The listing builds one solid part. Answer for the finished solid, in the listing's coordinates (mm). Face numbers are marked on the shaded views. Round coordinates to 2 decimals unless told otherwise and drop trailing zeros. Write each loop counter-clockwise with the first axis right and the second up, starting at its lowest first coordinate (ties: lowest second). Pieces come first, ordered by that corner, then holes. Notation, with made-up numbers: (-12, 34.25) - (34, 34.25) arc R6 ccw to (34, 44.25) - close; hole circle Ø1 at (-9.75, -8). An arc over 180 degrees is marked (long way). Answer as CSV lines item,"result". Start each with the question number.
Item 1: A cutting plane is placed at B-B on y = 0. Determine the outline of the cut face in (x, z), and give its area (3 significant figures).
Item 2: Straight lines are drawn through the part: line 1 along X through (y, z) = (0, 13.25); line 2 along Y through (x, z) = (25.5, -5); line 3 along Y through (x, z) = (-10.5, 2). For each, find the intervals that lie inside material, in ascending order. Write a range as [from, to].
Item 3: Flat-ended cylindrical pins translate along their axes: pin 1 (1.4 mm diameter, centred on x = -12, z = 9, fed in from +Y); pin 2 (3 mm diameter, centred on x = 29.337, y = 0, fed in from -Z); pin 3 (1 mm diameter, centred on x = -6, y = 12.5, fed in from -Z). Find the tip coordinate at first contact, or state that the pin passes through.
Item 4: A cutting plane is placed at A-A on z = 0. Determine the outline of the cut face in (x, y), and give its area (3 significant figures).
Item 5: For a pull along Z with two mould halves and no side action, classify the marked faces 1, 2 and 3 as pulls with the +Z half, pulls with the -Z half, needs draft (parallel to the pull), parting line crosses it, or undercut.
```python
from build123d import *

# Parameters (mm, degrees)
F0_R     = 19.05
F1_DEPTH = 42.037
F4_D     = 3.7973
F4_DEPTH = 12
F4_START = 0.0948523
F4_TIP   = 1.1408240143
F5_SIZE  = 1.524


with BuildPart() as f1:
    # F0 (on Right) → F1 (new body, symmetric)
    with BuildSketch(Plane.YZ):
        Circle(F0_R)
        with BuildLine():
            ThreePointArc((2.38125, 7.5718924112), (0, -7.9375), (-2.38125, 7.5718924112))
            Line((-2.38125, 7.5718924112), (-2.38125, 10.31875))
            Line((-2.38125, 10.31875), (2.38125, 10.31875))
            Line((2.38125, 10.31875), (2.38125, 7.5718924112))
        make_face(mode=Mode.SUBTRACT)
    extrude(amount=F1_DEPTH, both=True)

    # F4
    # its depths count from where the whole tool has entered the part; down to there all is cleared
    with Locations(Plane.XY.offset(19.05).offset(-F4_START)):
        with Locations((29.337, 0), (-29.337, 0)):
            Hole(F4_D / 2, depth=F4_DEPTH)
            with Locations((0, 0, -(F4_DEPTH + F4_TIP / 2))):  # 118° drill point
                Cone(0, F4_D / 2, F4_TIP, mode=Mode.SUBTRACT)

    # F5
    f5_edges = [f1.edges().sort_by_distance(p)[0] for p in [
        (42.037, -19.05, 0),
        (-42.037, -19.05, 0),
    ]]
    chamfer(f5_edges, length=F5_SIZE)


solid = f1.part
```
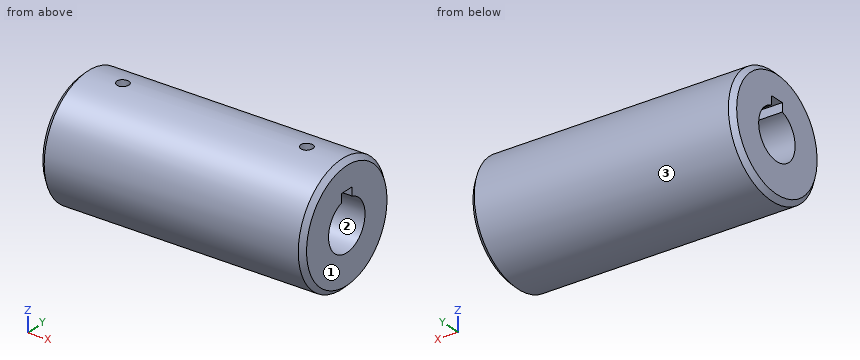
Geometry says:
1,outline,"(-42.04, -17.53) - (-40.51, -19.05) - (40.51, -19.05) - (42.04, -17.53) - (42.04, -7.94) - (-42.04, -7.94) - close; (-42.04, 10.32) - (-31.24, 10.32) - (-31.24, 19.05) - (-40.51, 19.05) - (-42.04, 17.53) - close; (-27.44, 10.32) - (27.44, 10.32) - (27.44, 19.05) - (-27.44, 19.05) - close; (31.24, 10.32) - (42.04, 10.32) - (42.04, 17.53) - (40.51, 19.05) - (31.24, 19.05) - close"
1,area,"1,600 mm^2"
2,line 1,"x = [-42.04, -31.24], [-27.44, 27.44], [31.24, 42.04]"
2,line 2,"y = [-18.38, -6.16], [6.16, 18.38]"
2,line 3,"y = [-18.94, -7.68], [7.68, 18.94]"
3,pin 1,"stops at y = 17.15"
3,pin 2,"stops at z = -19.05"
3,pin 3,"stops at z = -14.8"
4,outline,"(-42.04, -17.53) - (-40.51, -19.05) - (40.51, -19.05) - (42.04, -17.53) - (42.04, -7.94) - (-42.04, -7.94) - close; (-42.04, 7.94) - (42.04, 7.94) - (42.04, 17.53) - (40.51, 19.05) - (-40.51, 19.05) - (-42.04, 17.53) - close"
4,area,"1,860 mm^2"
5,face 1,"needs draft"
5,face 2,"undercut"
5,face 3,"parting line crosses it"
